```python
from build123d import *

# Parameters (mm, degrees)
F0_W           = 40
F0_H           = 15
F1_DEPTH       = 16
F2_R           = 5
F5_D           = 2.5
F5_DEPTH       = 7.4
F5_TIP         = 0.7510757738
F5_ON_F4_D     = 2.5
F5_ON_F4_DEPTH = 7.4
F5_ON_F4_TIP   = 0.7510757738


with BuildPart() as f1:
    # F0 (on Top) → F1 (new body)
    with BuildSketch(Plane.XY):
        Polygon((173.2976804376, -4.1842792928), (-85.7023195624, -4.1842792928), (-85.7023195624, -44.1842792928), (-45.7023195624, -44.1842792928), (133.2976804376, -44.1842792928), (173.2976804376, -44.1842792928), align=None)
        with Locations((-65.7023195624, -51.6842792928)):
            Rectangle(F0_W, F0_H)
        with Locations((153.2976804376, -51.6842792928)):
            Rectangle(F0_W, F0_H)
    extrude(amount=F1_DEPTH)

    # F2
    f2_edges = [f1.edges().sort_by_distance(p)[0] for p in [
        (-45.70232, -59.184279, 8),
        (133.29768, -59.184279, 8),
        (133.29768, -44.184279, 8),
        (-45.70232, -44.184279, 8),
    ]]
    fillet(f2_edges, radius=F2_R)

    # F5
    with Locations(Plane(origin=(-85.7023195624, 0, 0), x_dir=(0, -1, 0), z_dir=(-1, 0, 0))):
        with Locations((12.9342792928, 8), (55.4342792928, 8)):
            Hole(F5_D / 2, depth=F5_DEPTH)
            with Locations((0, 0, -(F5_DEPTH + F5_TIP / 2))):  # 118° drill point
                Cone(0, F5_D / 2, F5_TIP, mode=Mode.SUBTRACT)

    # F5 on F4
    with Locations(Plane.YZ.offset(173.2976804376)):
        with Locations((-12.9342792928, 8), (-55.4342792928, 8)):
            Hole(F5_ON_F4_D / 2, depth=F5_ON_F4_DEPTH)
            with Locations((0, 0, -(F5_ON_F4_DEPTH + F5_ON_F4_TIP / 2))):  # 118° drill point
                Cone(0, F5_ON_F4_D / 2, F5_ON_F4_TIP, mode=Mode.SUBTRACT)


solid = f1.part
```
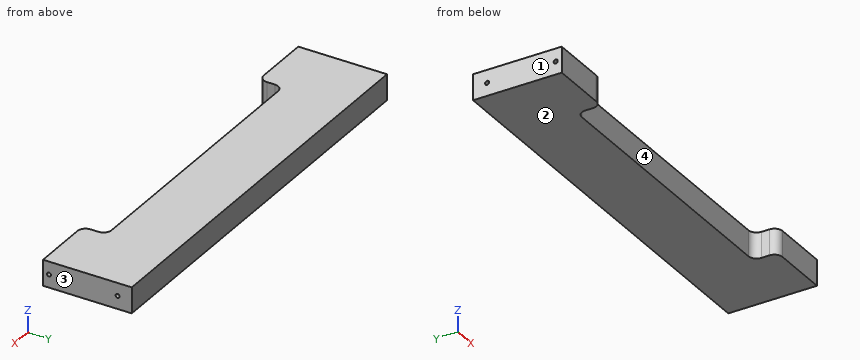
CAD build for the part. Positions are in the model's coordinates, mm. Face numbers are marked on the shaded views. Coordinates: 2 decimals unless noted, no trailing zeros. Order: outer loops, then holes, each group sorted by start corner. A loop starts at its lowest first (then second) coordinate and runs counter-clockwise, first axis right, second up. Notation, with made-up numbers: M -32.5,56 L -18.5,56 A24 cw -18.5,92 Z; hole C 56,-6 d4. An arc over 180 degrees is marked long. Write each question's results on one line, items separated by ' | '. Start each with the question number.
Q1. Cut at B-B (x = 77). List the corners of the cut face in (y, z).
Q2. Drill centre lines: probe 1 along Y at (x, z) = (-80.5, 8); probe 2 along X at (y, z) = (-49.5, 3.25); probe 3 along Y at (x, z) = (25, 8.5). Where is each one in solid material? Low to high. Write a range as from..to.
Q3. Pull direction X, two halves, no side cores. Call the marked faces 1, 2, 3 and 4: +X half, -X half, draft (parallel to the pull), parting line (faces both ways), or undercut.
Q4. Cut at A-A (z = 2.5). List the corners of the cut face in (x, y), then the cut area to 3 significant figures.
Found:
1) outline: M -44.18,0 L -4.18,0 L -4.18,16 L -44.18,16 Z
2) probe 1: -59.18..-56.68, -54.18..-14.18, -11.68..-4.18 | probe 2: -85.7..-45.7, 133.3..173.3 | probe 3: -44.18..-4.18
3) face 1: -X half | face 2: draft | face 3: +X half | face 4: undercut
4) outline: M -85.7,-59.18 L -50.7,-59.18 A5 ccw -45.7,-54.18 L -45.7,-49.18 A5 cw -40.7,-44.18 L 128.3,-44.18 A5 cw 133.3,-49.18 L 133.3,-54.18 A5 ccw 138.3,-59.18 L 173.3,-59.18 L 173.3,-4.18 L -85.7,-4.18 Z | area: 11,600 mm²
